Geometry check sheet. Reference: drawing and pictorial views, mm from the part's lowest x, y, z. Round coordinates to 2 decimals unless told otherwise and drop trailing zeros. Order: outer loops, then holes, each group sorted by start corner. A loop starts at its lowest first (then second) coordinate and runs counter-clockwise, first axis right, second up.
Q1. Cross-section at C-C on y = 22. Record the cut outline in (x, z).
Q2. Scan lines: probe 1 along Y at (x, z) = (58.5, 85); probe 2 along X at (y, z) = (4, 50); probe 3 along Z at (x, y) = (24.5, 7.25) (1 decimal). Record each from-to range of solid material in increasing order.
Q3. Depth check by flat-ended pin: P1, Ø1, axis at y = 7, z = 169.5, coming from the +X side; P2, Ø4, axis at x = 173, z = 67, coming from the -Y side; P3, Ø5, axis at x = 23.5, y = 24.5, coming from the -Z side; P4, Ø8, axis at x = 56, y = 17, coming from the -Z side. Enter the tip coordinate at first touch or a pass-through.
Q4. Cross-section at B-B on x = 96. Record the cut outline in (y, z).
Q5. Cross-section at A-A on z = 100. Record the cut outline in (x, y).
Q6. Mould release check, pull along Z, two halves, no side actions. Record for the marked faces 1, 2, 3 and 4: +Z half, -Z half, draft (parallel to the pull), parting line (faces both ways), or undercut.
Q7. Cross-section at D-D on z = 50. Record the cut outline in (x, y), then the cut area to 3 significant figures.
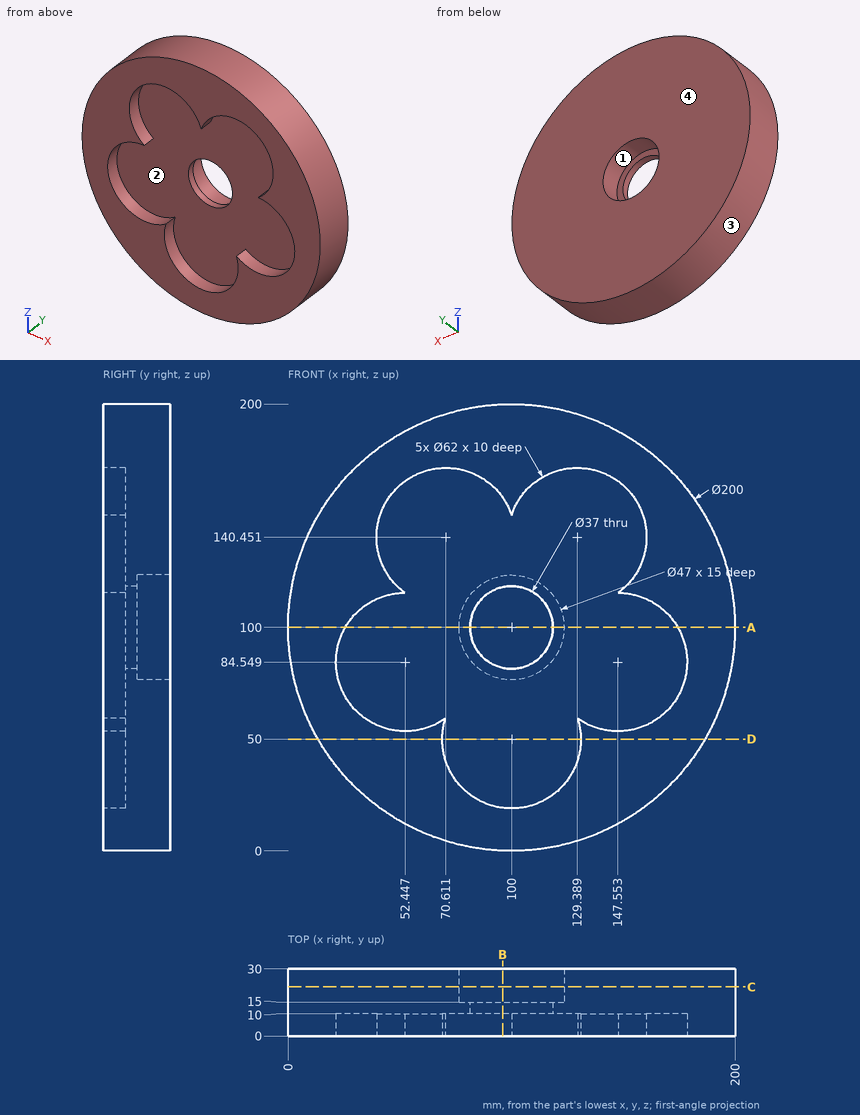
Results found:
1. outline: circle Ø200 at (100, 100); hole circle Ø47 at (100, 100)
2. probe 1: y = 10 to 30
2. probe 2: x = 13.4 to 69, 131 to 186.6
2. probe 3: z = 34.4 to 71.1, 98 to 165.6
3. P1: stops at x = 172.38
3. P2: stops at y = 0
3. P3: stops at z = 32.74
3. P4: stops at z = 8.35
4. outline: (0, 0.08) - (30, 0.08) - (30, 76.84) - (15, 76.84) - (15, 81.94) - (10, 81.94) - (10, 19.26) - (0, 19.26) - close; (0, 158.24) - (10, 158.24) - (10, 118.06) - (15, 118.06) - (15, 123.16) - (30, 123.16) - (30, 199.92) - (0, 199.92) - close
5. outline: (0, 0) - (25.57, 0) - (25.57, 10) - (81.5, 10) - (81.5, 15) - (76.5, 15) - (76.5, 30) - (0, 30) - close; (118.5, 10) - (174.43, 10) - (174.43, 0) - (200, 0) - (200, 30) - (123.5, 30) - (123.5, 15) - (118.5, 15) - close
6. face 1: undercut
6. face 2: undercut
6. face 3: parting line
6. face 4: draft
7. outline: (13.4, 0) - (69, 0) - (69, 10) - (131, 10) - (131, 0) - (186.6, 0) - (186.6, 30) - (13.4, 30) - close
7. area: 4,580 mm2
